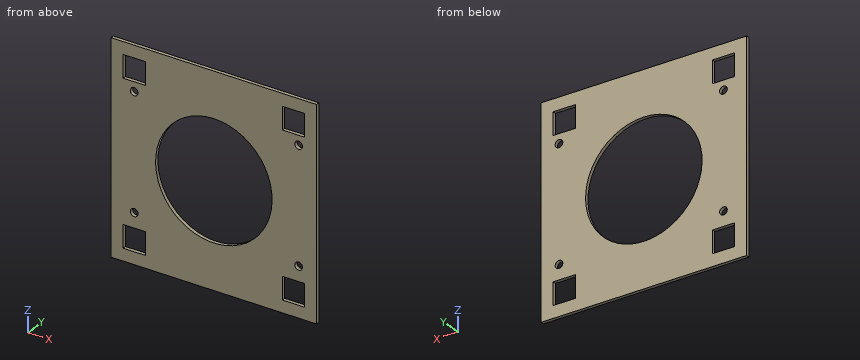
from build123d import *

# Parameters (mm, degrees)
SKETCH1_W           = 381
SKETCH1_H           = 381
BOSS_EXTRUDE1_DEPTH = 6.35
SKETCH2_R           = 107.95
CUT_EXTRUDE1_DEPTH  = 6.35
SKETCH3_W           = 41.148
SKETCH3_H           = 41.148
CUT_EXTRUDE2_DEPTH  = 6.35
SKETCH3_4_R         = 7.112
CUT_EXTRUDE3_DEPTH  = 270.482508709


with BuildPart() as part:
    # Sketch1 → Boss-Extrude1 (new body)
    with BuildSketch(Plane(origin=(0, 0, 0), x_dir=(1, 0, 0), z_dir=(0, 1, 0))):
        Rectangle(SKETCH1_W, SKETCH1_H)
    extrude(amount=BOSS_EXTRUDE1_DEPTH)

    # Sketch2 → Cut-Extrude1 (cut)
    with BuildSketch(Plane(origin=(0, 6.35, 0), x_dir=(1, 0, 0), z_dir=(0, 1, 0))):
        with Locations(Location((0, 0, 0), (0, 0, 270))):
            Circle(SKETCH2_R)
    extrude(amount=-CUT_EXTRUDE1_DEPTH, mode=Mode.SUBTRACT)

    # Sketch3 → Cut-Extrude2 (cut)
    with BuildSketch(Plane(origin=(0, 6.35, 0), x_dir=(1, 0, 0), z_dir=(0, 1, 0))):
        with Locations((-147.574, 147.574)):
            Rectangle(SKETCH3_W, SKETCH3_H)
        with Locations((147.574, 147.574)):
            Rectangle(SKETCH3_W, SKETCH3_H)
        with Locations((147.574, -147.574)):
            Rectangle(SKETCH3_W, SKETCH3_H)
        with Locations((-147.574, -147.574)):
            Rectangle(SKETCH3_W, SKETCH3_H)
    extrude(amount=-CUT_EXTRUDE2_DEPTH, mode=Mode.SUBTRACT)

    # Sketch3_4 → Cut-Extrude3 (cut, through all)
    with BuildSketch(Plane(origin=(0, 6.35, 0), x_dir=(1, 0, 0), z_dir=(0, 1, 0))):
        with Locations(Location((157.226, 100.076, 0), (0, 0, 270))):
            Circle(SKETCH3_4_R)
        with Locations(Location((-147.574, -109.728, 0), (0, 0, 270))):
            Circle(SKETCH3_4_R)
        with Locations(Location((-147.574, 100.076, 0), (0, 0, 270))):
            Circle(SKETCH3_4_R)
        with Locations(Location((157.226, -109.728, 0), (0, 0, 270))):
            Circle(SKETCH3_4_R)
    extrude(amount=-CUT_EXTRUDE3_DEPTH, mode=Mode.SUBTRACT)


solid = part.part
Work out the finished part from the listing and answer in its coordinate system (mm). Coordinates: 2 decimals unless noted, no trailing zeros. Write each loop counter-clockwise with the first axis right and the second up, starting at its lowest first coordinate (ties: lowest second). Pieces come first, ordered by that corner, then holes. Notation, with made-up numbers: (19.5, 12.5) - (33.5, 12.5) arc R29 ccw to (33.5, 39.5) - close; hole circle Ø11 at (36.5, 15.5). An arc over 180 degrees is marked (long way). One line per question, with ' | ' between items.
1) A flat-ended cylindrical pin translates along its axis: P1, Ø23, axis at x = 157.226, z = 109.728, coming from the -Y side. Find the tip coordinate at first contact, or state that the pin passes through.
Checks:
P1: y = 0
2) Find section A-A, the plane x = 0. Determine the outline of the cut face in (y, z), and give its area (3 significant figures).
Checks:
outline: (0, -190.5) - (6.35, -190.5) - (6.35, -107.95) - (0, -107.95) - close; (0, 107.95) - (6.35, 107.95) - (6.35, 190.5) - (0, 190.5) - close | area: 1,050 mm2
3) Find section B-B, the plane z = 0. Determine the outline of the cut face in (x, y), and give its area (3 significant figures).
Checks:
outline: (-190.5, 0) - (-107.95, 0) - (-107.95, 6.35) - (-190.5, 6.35) - close; (107.95, 0) - (190.5, 0) - (190.5, 6.35) - (107.95, 6.35) - close | area: 1,050 mm2
4) Find section D-D, the plane y = 4.75. Give the number of separate pieces and of enclosed holes in the cut face, and give its area (3 significant figures).
Checks:
separate pieces: 1 | enclosed holes: 9 | area: 101,000 mm2
5) Find section C-C, the plane x = 138.5. Determine the outline of the cut face in (y, z).
Checks:
outline: (0, -190.5) - (6.35, -190.5) - (6.35, -168.15) - (0, -168.15) - close; (0, -127) - (6.35, -127) - (6.35, 127) - (0, 127) - close; (0, 168.15) - (6.35, 168.15) - (6.35, 190.5) - (0, 190.5) - close
6) Consider probe 1 along X at (y, z) = (5.75, 157); probe 2 along X at (y, z) = (1.5, 0); probe 3 along Z at (x, y) = (-149.5, 0.5). Determine where each line is inside the solid, lowest interval first. Write a range as [from, to].
Checks:
probe 1: [-190.5, -168.15], [-127, 127], [168.15, 190.5] | probe 2: [-190.5, -107.95], [107.95, 190.5] | probe 3: [-190.5, -168.15], [-127, -106.92], [-93.23, 102.88], [116.57, 127], [168.15, 190.5]
